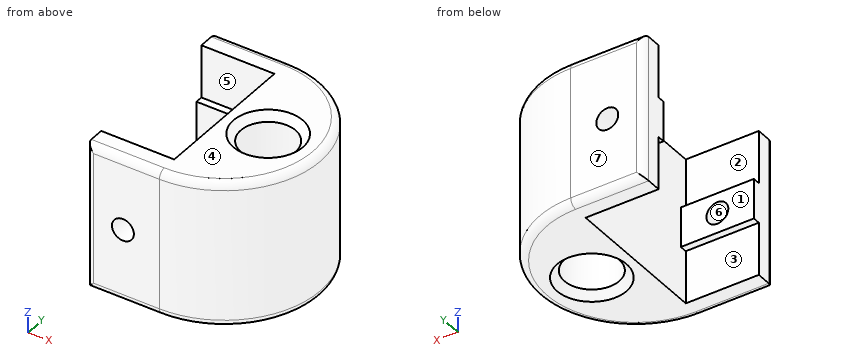
```python
from build123d import *

# Parameters (mm, degrees)
F0_R     = 3.75
F1_DEPTH = 20
F2_W     = 1
F2_H     = 5.5
F3_DEPTH = 10
F4_R     = 1.5
F5_DEPTH = 26.301
F6_SIZE  = 1
F7_R     = 1


with BuildPart() as f1:
    # F0 (on Top) → F1 (new body)
    with BuildSketch(Plane.XY):
        with BuildLine():
            Line((0, 3), (0, 0))
            Line((0, 0), (10, 0))
            ThreePointArc((10, 0), (23.15, 13.15), (10, 26.3))
            Line((10, 26.3), (0, 26.3))
            Line((0, 26.3), (0, 23.3))
            Line((0, 23.3), (10, 23.3))
            Line((10, 23.3), (10, 3))
            Line((10, 3), (0, 3))
        make_face()
        with Locations((16, 13.15)):
            Circle(F0_R, mode=Mode.SUBTRACT)
    extrude(amount=F1_DEPTH)

    # F2 (on face) → F3 (join, through all)
    with BuildSketch(Plane(origin=(10, 0, 0), x_dir=(0, -1, 0), z_dir=(-1, 0, 0))):
        with Locations((-22.8, 10)):
            Rectangle(F2_W, F2_H)
        with Locations((-3.5, 10)):
            Rectangle(F2_W, F2_H)
    extrude(amount=F3_DEPTH)

    # F4 (on face) → F5 (cut, through all)
    with BuildSketch(Plane.XZ):
        with Locations((5, 10)):
            Circle(F4_R)
    extrude(amount=-F5_DEPTH, mode=Mode.SUBTRACT)

    # F6
    f6_edges = [f1.edges().sort_by_distance(p)[0] for p in [
        (12.25, 13.15, 20),
        (12.25, 13.15, 0),
    ]]
    chamfer(f6_edges, length=F6_SIZE)

    # F7
    f7_edges = [f1.edges().sort_by_distance(p)[0] for p in [
        (23.15, 13.15, 20),
        (23.15, 13.15, 0),
        (0, 0, 10),
        (0, 26.3, 10),
    ]]
    fillet(f7_edges, radius=F7_R)


solid = f1.part
```
Input: part model. Units: mm. Frame: model coordinates. Face numbers are marked on the shaded views. A direction names the side the tool comes from. Round coordinates to 2 decimals unless told otherwise and drop trailing zeros. Loops run counter-clockwise (first coordinate to the right, second up) from the corner with the lowest first, then second, coordinate; pieces in that order, holes last. Notation, with made-up numbers: M -5,61.25 L 20,61.25 A12 ccw 20,82.25 Z; hole C -18,-14 d4. An arc over 180 degrees is marked long. Answer in a Markdown table with one row per item. Add a question column.
1. Section A-A (z = 10). Output: boundary loops of the cut face in (x, y), and give its area (3 significant figures).
2. Contact query for flat-ended pins moving along their axis: pin 1 (6 mm diameter, centred on y = 8, z = 4.5, fed in from +X); pin 2 (0.8 mm diameter, centred on x = 7, y = 23, fed in from +Z); pin 3 (3 mm diameter, centred on y = 16, z = 13, fed in from -X); pin 4 (6 mm diameter, centred on x = 17.5, z = 13, fed in from -Y). Output: stop coordinate, or through.
3. Section C-C (x = 5). Output: boundary loops of the cut face in (y, z), and give its area (3 significant figures).
4. Section D-D (y = 13.15). Output: boundary loops of the cut face in (x, z), and give its area (3 significant figures).
5. Mould query, pull axis Y, two halves, no side actions, for the marked faces 5, 6 and 7. Classes: released by +Y, released by -Y, zero draft, split by the parting line, or undercut.
6. Section B-B (x = 8). Output: boundary loops of the cut face in (y, z).
7. Set-up query: the marked faces 1, 2, 3 and 4. Return all of +Z, -Z, +X, -X, +Y, -Y with unobstructed straight access to the full face (end or side cutting, diameter ignored); none if empty.
8. Ray query, probe 1 along Y at (x, z) = (8.5, 6.5); probe 2 along Z at (x, y) = (5, 24.8); probe 3 along Z at (x, y) = (5, 3.15). Return the intervals inside material, ascending.
Values follow:
| question | item | result |
|---|---|---|
| 1 | outline | M 0,1 A1 ccw 1,0 L 3.5,0 L 3.5,4 L 0,4 Z; M 0,22.3 L 3.5,22.3 L 3.5,26.3 L 1,26.3 A1 ccw 0,25.3 Z; M 6.5,0 L 10,0 A13.15 ccw 10,26.3 L 6.5,26.3 L 6.5,22.3 L 10,22.3 L 10,4 L 6.5,4 Z; hole C 16,13.15 d7.5 |
| 1 | area | 283 mm^2 |
| 2 | pin 1 | x = 22.97 |
| 2 | pin 2 | z = 20 |
| 2 | pin 3 | x = 10 |
| 2 | pin 4 | y = 0.79 |
| 3 | outline | M 0,1 A1 ccw 1,0 L 3,0 L 3,7.25 L 4,7.25 L 4,8.5 L 0,8.5 Z; M 0,11.5 L 4,11.5 L 4,12.75 L 3,12.75 L 3,20 L 1,20 A1 ccw 0,19 Z; M 22.3,7.25 L 23.3,7.25 L 23.3,0 L 25.3,0 A1 ccw 26.3,1 L 26.3,8.5 L 22.3,8.5 Z; M 22.3,11.5 L 26.3,11.5 L 26.3,19 A1 ccw 25.3,20 L 23.3,20 L 23.3,12.75 L 22.3,12.75 Z |
| 3 | area | 106 mm^2 |
| 4 | outline | M 10,0 L 11.25,0 L 12.25,1 L 12.25,19 L 11.25,20 L 10,20 Z; M 19.75,1 L 20.75,0 L 22.15,0 A1 ccw 23.15,1 L 23.15,19 A1 ccw 22.15,20 L 20.75,20 L 19.75,19 Z |
| 4 | area | 111 mm^2 |
| 5 | face 5 | undercut |
| 5 | face 6 | zero draft |
| 5 | face 7 | released by +Y |
| 6 | outline | M 0,1 A1 ccw 1,0 L 3,0 L 3,7.25 L 4,7.25 L 4,12.75 L 3,12.75 L 3,20 L 1,20 A1 ccw 0,19 Z; M 22.3,7.25 L 23.3,7.25 L 23.3,0 L 25.3,0 A1 ccw 26.3,1 L 26.3,19 A1 ccw 25.3,20 L 23.3,20 L 23.3,12.75 L 22.3,12.75 Z |
| 7 | face 1 | +Z, -Z, -X |
| 7 | face 2 | +Z, -X |
| 7 | face 3 | -Z, -X |
| 7 | face 4 | +Z, +X, -X, +Y, -Y |
| 8 | probe 1 | 0 to 3, 23.3 to 26.3 |
| 8 | probe 2 | 0 to 8.5, 11.5 to 20 |
| 8 | probe 3 | 7.25 to 8.5, 11.5 to 12.75 |
